Here's the drawing with two shaded views (mm, measured from the low corner). I have some questions. A direction names the side the tool comes from. Round coordinates to 2 decimals unless told otherwise and drop trailing zeros. Write each loop counter-clockwise with the first axis right and the second up, starting at its lowest first coordinate (ties: lowest second). Pieces come first, ordered by that corner, then holes. Notation, with made-up numbers: M 36.25,-4 L 78.25,-4 A18 cw 78.25,17 Z; hole C 55,61 d5. An arc over 180 degrees is marked long. Answer as a JSON object with one key per item and string values. Group by question number.
1) Suppose I cut it at B-B, the plane x = 3.9. Write out the boundary of the cut face in (y, z).
2) Please list where these lines run through material, in increasing order: L1, parallel to Z at x = 10.5, y = 2.3; L2, parallel to Y at x = 16.75, z = 13.75; L3, parallel to Y at x = 9.5, z = 1. Write a range as [from, to].
3) On a 3-axis mill with a long thin cutter (end or side, diameter ignored), from which of +Z, -Z, +X, -X, +Y, -Y can I reach the whole of each face in a straight line? I mean the marked faces 1 and 2. Say none if no direction works.
4) If we mould it in two halves opening along X, with no side actions, what happens to the marked faces 3, 4, 5 and 6? For each: +X half, -X half, draft (parallel to the pull), parting line (faces both ways), or undercut.
5) Suppose I cut it at D-D, the plane x = 10.25. Write out the boundary of the cut face in (y, z), and give its area (3 significant figures).
6) Suppose I cut it at A-A, the plane z = 13. Write out the boundary of the cut face in (x, y).
7) Suppose I cut it at C-C, the plane x = 7. Write out the boundary of the cut face in (y, z).
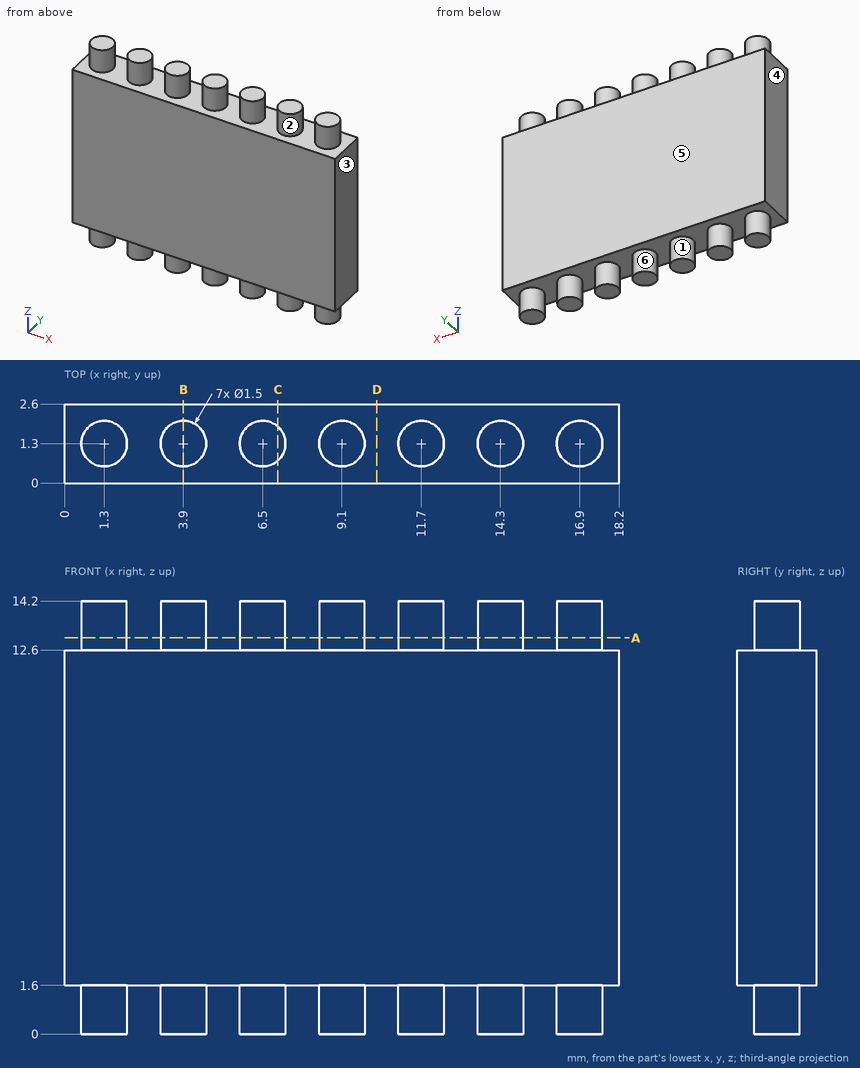
Results:
{
 "1": {"outline": "M 0,1.6 L 0.55,1.6 L 0.55,0 L 2.05,0 L 2.05,1.6 L 2.6,1.6 L 2.6,12.6 L 2.05,12.6 L 2.05,14.2 L 0.55,14.2 L 0.55,12.6 L 0,12.6 Z"},
 "2": {"L1": "[1.6, 12.6]", "L2": "[0.57, 2.03]", "L3": "[0.67, 1.93]"},
 "3": {"face 1": "-Z", "face 2": "+Z"},
 "4": {"face 3": "+X half", "face 4": "-X half", "face 5": "draft", "face 6": "undercut"},
 "5": {"outline": "M 0,1.6 L 2.6,1.6 L 2.6,12.6 L 0,12.6 Z", "area": "28.6 mm^2"},
 "6": {"outline": "C 1.3,1.3 d1.5; C 3.9,1.3 d1.5; C 6.5,1.3 d1.5; C 9.1,1.3 d1.5; C 11.7,1.3 d1.5; C 14.3,1.3 d1.5; C 16.9,1.3 d1.5"},
 "7": {"outline": "M 0,1.6 L 0.74,1.6 L 0.74,0 L 1.86,0 L 1.86,1.6 L 2.6,1.6 L 2.6,12.6 L 1.86,12.6 L 1.86,14.2 L 0.74,14.2 L 0.74,12.6 L 0,12.6 Z"}
}
